from build123d import *

# Parameters (mm, degrees)
SKETCH2_R          = 2.413
CUT_EXTRUDE1_DEPTH = 99.425
CIRPATTERN1_COUNT  = 6


with BuildPart() as part:
    # Sketch1 → Revolve1 (revolve)
    with BuildSketch(Plane.XY):
        Polygon((96.8375, 0), (96.8375, 12.7), (98.425, 12.7), (98.425, -0.383318861), (34.307471211, -125.4125), (33.3375, -125.4125), (33.3375, -123.825), align=None)
    revolve(axis=Axis((0, 0, 0), (0, -1, 0)))

    # Sketch2 → Cut-Extrude1 (cut, symmetric)
    with BuildSketch(Plane.XY):
        with Locations((0, 6.35)):
            Circle(SKETCH2_R)
    cut_extrude1 = extrude(amount=CUT_EXTRUDE1_DEPTH, both=True, mode=Mode.SUBTRACT)

    # CirPattern1: Cut-Extrude1 ×6 about axis
    cirpattern1_axis = Axis((0, 12.7, 0), (0, 1, 0))
    for i in range(1, CIRPATTERN1_COUNT):
        add(cut_extrude1.rotate(cirpattern1_axis, i * 360 / CIRPATTERN1_COUNT), mode=Mode.SUBTRACT)


solid = part.part
Here's how the part is built. I have some questions about the finished solid (model axes, mm). A direction names the side the tool comes from. Coordinates: 2 decimals unless noted, no trailing zeros. Order: outer loops, then holes, each group sorted by start corner. A loop starts at its lowest first (then second) coordinate and runs counter-clockwise, first axis right, second up.
Item 1: If we mould it in two halves opening along Y, with no side actions, what happens to faces 3 (the face through (-0.314, 8.742, 97.628)), 4 (the face through (31.8, -124.61, 10.01)), 5 (the face through (-5.2, -125.412, 33.2)), 6 (the face through (-72, 12.7, -65))? For each: +Y half, -Y half, draft (parallel to the pull), parting line (faces both ways), or undercut.
Result sheet:
face 3: undercut
face 4: draft
face 5: -Y half
face 6: +Y half
Item 2: I need wall thicknesses on line 1 (Z direction, x = 0, y = 2.5) (1 decimal); line 2 (Z direction, x = -11, y = -43); line 3 (X direction, y = -69, z = 48.5). Which ranges of each line are inside material? Lowest first, please.
Result sheet:
line 1: z = -98.4 to -96.8, 96.8 to 98.4
line 2: z = -75.78 to -73.97, 73.97 to 75.78
line 3: x = -40.58 to -37.74, 37.74 to 40.58
Item 3: For P1, Ø4, axis at x = 11, z = -36.5, coming from the +Y side; P2, Ø1.5, axis at y = -63, z = 4, coming from the -X side; P3, Ø6, axis at x = 30.5, z = 66, coming from the +Y side, each with a flat end and sliding along its axis, tell me the tip position at first contact or that it passes through.
Result sheet:
P1: stops at y = -110.6
P2: stops at x = -66.58
P3: stops at y = -41.21
Item 4: If we section it at A-A on z = 0: List the corners of the cut face in (x, y) for me (1 decimal).
Result sheet:
outline: (-98.4, -0.4) - (-34.3, -125.4) - (-33.3, -125.4) - (-33.3, -123.8) - (-96.8, 0) - (-96.8, 12.7) - (-98.4, 12.7) - close; (33.3, -125.4) - (34.3, -125.4) - (98.4, -0.4) - (98.4, 12.7) - (96.8, 12.7) - (96.8, 0) - (33.3, -123.8) - close
Item 5: For faces 1 (the face through (-0.314, 8.742, -97.605)), 2 (the face through (-20.992, 6.439, -94.535)), which set-ups out of +Z, -Z, +X, -X, +Y, -Y let a thin tool reach every point of the face, with its end or its side?
Result sheet:
face 1: +Z, -Z
face 2: +Y
Item 6: If we section it at B-B on y = -9: List the corners of the cut face in (x, z) for me.
Result sheet:
outline: circle Ø188.01 at (0, 0); hole circle Ø184.44 at (0, 0)
Item 7: If we section it at C-C on y = -112.5: List the corners of the cut face in (x, z) for me.
Result sheet:
outline: circle Ø81.86 at (0, 0); hole circle Ø78.29 at (0, 0)
